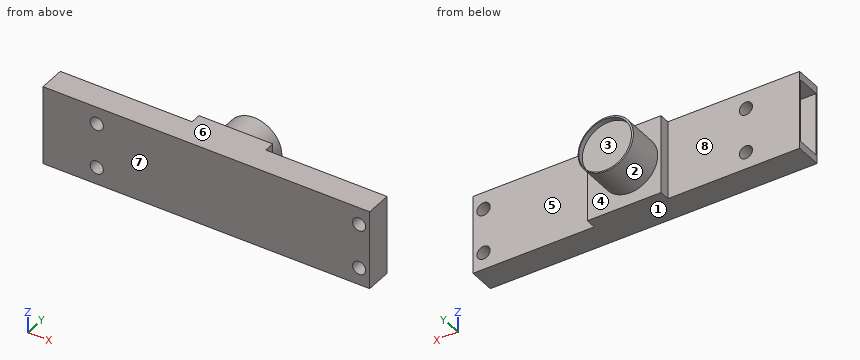
```python
from build123d import *

# Parameters (mm, degrees)
SKETCH1_W           = 62
SKETCH1_H           = 15
SKETCH1_R           = 5.25
BOSS_EXTRUDE1_DEPTH = 5
SKETCH1_7_R         = 1.25
CUT_EXTRUDE1_DEPTH  = 5
SKETCH1_8_W         = 14
SKETCH1_8_H         = 15
BOSS_EXTRUDE2_DEPTH = 7
SKETCH1_9_R         = 5.25
BOSS_EXTRUDE3_DEPTH = 14
SKETCH2_R           = 5
CUT_EXTRUDE2_DEPTH  = 1
SKETCH3_W           = 12
SKETCH3_H           = 4.5
CUT_EXTRUDE4_DEPTH  = 8


with BuildPart() as part:
    # Sketch1 → Boss-Extrude1 (new body)
    with BuildSketch(Plane(origin=(0, 0, 0), x_dir=(1, 0, 0), z_dir=(0, 1, 0))):
        Rectangle(SKETCH1_W, SKETCH1_H)
        with Locations(Location((-0.12, 0, 0), (0, 0, 270))):
            Circle(SKETCH1_R, mode=Mode.SUBTRACT)
    extrude(amount=BOSS_EXTRUDE1_DEPTH)

    # Sketch1_7 → Cut-Extrude1 (cut)
    with BuildSketch(Plane(origin=(0, 0, 0), x_dir=(1, 0, 0), z_dir=(0, 1, 0))):
        with Locations(Location((29, 4.25, 0), (0, 0, 270))):
            Circle(SKETCH1_7_R)
        with Locations(Location((29, -4.25, 0), (0, 0, 270))):
            Circle(SKETCH1_7_R)
        with Locations(Location((-20.8, 4.25, 0), (0, 0, 270))):
            Circle(SKETCH1_7_R)
        with Locations(Location((-20.8, -4.25, 0), (0, 0, 270))):
            Circle(SKETCH1_7_R)
    extrude(amount=CUT_EXTRUDE1_DEPTH, mode=Mode.SUBTRACT)

    # Sketch1_8 → Boss-Extrude2 (add)
    with BuildSketch(Plane(origin=(0, 0, 0), x_dir=(1, 0, 0), z_dir=(0, 1, 0))):
        with Locations((1, 0)):
            Rectangle(SKETCH1_8_W, SKETCH1_8_H)
    extrude(amount=BOSS_EXTRUDE2_DEPTH)

    # Sketch1_9 → Boss-Extrude3 (add)
    with BuildSketch(Plane(origin=(0, 0, 0), x_dir=(1, 0, 0), z_dir=(0, 1, 0))):
        with Locations(Location((-0.12, 0, 0), (0, 0, 270))):
            Circle(SKETCH1_9_R)
    extrude(amount=BOSS_EXTRUDE3_DEPTH)

    # Sketch2 → Cut-Extrude2 (cut)
    with BuildSketch(Plane(origin=(0, 14, 0), x_dir=(1, 0, 0), z_dir=(0, 1, 0))):
        with Locations(Location((0, 0, 0), (0, 0, 270))):
            Circle(SKETCH2_R)
    extrude(amount=-CUT_EXTRUDE2_DEPTH, mode=Mode.SUBTRACT)

    # Sketch3 → Cut-Extrude4 (cut)
    with BuildSketch(Plane.ZY.offset(31)):
        with Locations((0, 2.5)):
            Rectangle(SKETCH3_W, SKETCH3_H)
    extrude(amount=-CUT_EXTRUDE4_DEPTH, mode=Mode.SUBTRACT)


solid = part.part
```
Can you work these out from the model? Positions are in its coordinate system, mm. Face numbers are marked on the shaded views. A direction names the side the tool comes from. Give positions to 0.01 mm unless a question says otherwise; leave off trailing zeros. Write each loop counter-clockwise with the first axis right and the second up, starting at its lowest first coordinate (ties: lowest second). Pieces come first, ordered by that corner, then holes. Notation, with made-up numbers: (80, 24.5) -> (102, 24.5) arc R17 ccw to (102, 43.5) -> close; hole circle Ø5 at (-32, 70). An arc over 180 degrees is marked (long way). Write item = value, one per line.
(1) Thinking about a two-plate mould opening in X: for the marked faces 1, 2 and 3, which applies, released by +X, released by -X, zero draft, split by the parting line, or undercut?
Worked out:
face_1 = zero draft
face_2 = split by the parting line
face_3 = undercut
(2) For the marked faces 4, 5, 6, 7 and 8, which set-ups out of +Z, -Z, +X, -X, +Y, -Y let a thin tool reach every point of the face, with its end or its side?
Worked out:
face_4 = +Y
face_5 = +Z, -Z, +X, +Y
face_6 = +Z, +X, -X, +Y, -Y
face_7 = +Z, -Z, +X, -X, -Y
face_8 = +Z, -Z, -X, +Y
(3) Suppose I cut it at D-D on z = 4.25. Write out the boundary of the cut face in (x, y).
Worked out:
outline = (-31, 0) -> (-22.05, 0) -> (-22.05, 5) -> (-31, 5) -> (-31, 4.75) -> (-23, 4.75) -> (-23, 0.25) -> (-31, 0.25) -> close; (-19.55, 0) -> (27.75, 0) -> (27.75, 5) -> (8, 5) -> (8, 7) -> (2.96, 7) -> (2.96, 14) -> (2.63, 14) -> (2.63, 13) -> (-2.63, 13) -> (-2.63, 14) -> (-3.2, 14) -> (-3.2, 7) -> (-6, 7) -> (-6, 5) -> (-19.55, 5) -> close; (30.25, 0) -> (31, 0) -> (31, 5) -> (30.25, 5) -> close
(4) Suppose I cut it at A-A on y = 4. Write out the boundary of the cut face in (x, z), then the cut area to 3 significant figures.
Worked out:
outline = (-31, -7.5) -> (31, -7.5) -> (31, 7.5) -> (-31, 7.5) -> (-31, 6) -> (-23, 6) -> (-23, -6) -> (-31, -6) -> close; hole circle Ø2.5 at (-20.8, -4.25); hole circle Ø2.5 at (-20.8, 4.25); hole circle Ø2.5 at (29, -4.25); hole circle Ø2.5 at (29, 4.25)
area = 814 mm^2
(5) I need wall thicknesses on probe 1 along X at (y, z) = (2.5, -4.25); probe 2 along X at (y, z) = (2.5, 3.75); probe 3 along Y at (x, z) = (14.5, -1). Which ranges of each line are inside material? Lowest first, please. Write a range as from..to.
Worked out:
probe_1 = -23..-22.05, -19.55..27.75, 30.25..31
probe_2 = -23..-21.95, -19.65..27.85, 30.15..31
probe_3 = 0..5
(6) I'm going to push flat-ended pins straight in: P1, Ø5, axis at x = 0.5, z = -1, coming from the +Y side; P2, Ø4, axis at x = -20.8, z = 4.25, coming from the +Y side; P3, Ø8, axis at y = 12, z = -4.5, coming from the -X side. Where does each tip first touch, or does it pass through?
Worked out:
P1 = 13
P2 = 5
P3 = -5.35
(7) Suppose I cut it at B-B on x = -26. Write out the boundary of the cut face in (y, z), then the cut area to 3 significant figures.
Worked out:
outline = (0, -7.5) -> (5, -7.5) -> (5, 7.5) -> (0, 7.5) -> close; hole (0.25, -6) -> (4.75, -6) -> (4.75, 6) -> (0.25, 6) -> close
area = 21.0 mm^2
(8) Suppose I cut it at C-C on x = 29. Write out the boundary of the cut face in (y, z), then the cut area to 3 significant figures.
Worked out:
outline = (0, -7.5) -> (5, -7.5) -> (5, -5.5) -> (0, -5.5) -> close; (0, -3) -> (5, -3) -> (5, 3) -> (0, 3) -> close; (0, 5.5) -> (5, 5.5) -> (5, 7.5) -> (0, 7.5) -> close
area = 50.0 mm^2
